Autodesk Inventor part; units mm, degrees
ref_plane "Arbeitsebene1" through (0, 4, 0) normal (0, 1, 0) x (-1, 0, 0)
ref_plane "YZ Plane" through (0, 0, 0) normal (1, 0, 0) x (0, 1, 0)
ref_plane "XZ Plane" through (0, 0, 0) normal (0, 1, 0) x (-1, 0, 0)
sketch "Skizze1" plane through (0, 0, 0) normal (0, 0, 1) x (1, 0, 0)
  circle A0 centre (0, 0) radius 4
  point P0 (0, 4)
  dimension "d0" = 8
extrude "Extrusion1" add sketch "Skizze1" along normal blind 15
ref_plane "Arbeitsebene1" through (0, 4, 0) normal (0, 1, 0) x (-1, 0, 0)
sketch "Skizze2" plane through (0, 4, 0) normal (0, 1, 0) x (-1, 0, 0)
  point P0 (0, 0)
  point P1 (0, 7.5)
  dimension "d3" = 7.5
hole "Bohrung1" at (0, 4, 7.5) direction (0, -1, 0) diameter 3.242 end through all
chamfer "Fase1" distance 1 angle 45 2 edges at (-4, 0, 0) (-4, 0, 15)
properties part number "LANGMUTTER"
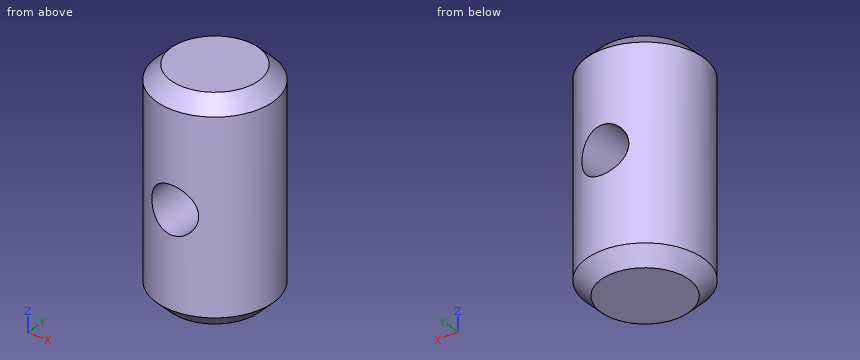
For this review, take the finished solid that the model builds, in its own axes (mm). Give positions to 0.01 mm unless a question says otherwise; leave off trailing zeros. Write each loop counter-clockwise with the first axis right and the second up, starting at its lowest first coordinate (ties: lowest second). Pieces come first, ordered by that corner, then holes. Notation, with made-up numbers: (-20, 66.5) -> (37, 66.5) arc R31 cw to (37, 91.5) -> close; hole circle Ø11 at (-13.75, 87.25). An arc over 180 degrees is marked (long way). Use CSV: the item, a comma, the result in double quotes.
Q1. To check wall thickness, follow probe 1 along Z at (x, y) = (0, -1.25); probe 2 along X at (y, z) = (-0.5, 7.5); probe 3 along Z at (x, y) = (1.25, 2). State the ranges of each line that lie inside material, in increasing order. Write a range as [from, to].
Conclusion:
probe 1,"[0, 5.88], [9.12, 15]"
probe 2,"[-3.97, -1.62], [1.62, 3.97]"
probe 3,"[0, 6.47], [8.53, 15]"
Q2. Take a section at C-C, the plane z = 6.5. Write out the cut boundary in (x, y).
Conclusion:
outline,"(-1.28, -3.79) -> (-1.28, 3.79) arc R4 ccw to start; (1.28, -3.79) arc R4 ccw to (1.28, 3.79) -> close"
Q3. Take a section at D-D, the plane z = 13.5. Write out the cut boundary in (x, y).
Conclusion:
outline,"circle Ø8 at (0, 0)"
Q4. For P1, Ø3, axis at y = -2, z = 13, coming from the +X side; P2, Ø2, axis at x = 2, z = 5, coming from the -Y side; P3, Ø1.5, axis at x = -3, z = 12.5, coming from the -Y side, all flat-tipped, find the tip position at first contact; note any pin that passes through.
Conclusion:
P1,"x = 3.97"
P2,"y = -3.87"
P3,"y = -3.31"
Q5. Take a section at B-B, the plane y = 0. Write out the cut boundary in (x, z), then the cut area to 3 significant figures.
Conclusion:
outline,"(-4, 1) -> (-3, 0) -> (3, 0) -> (4, 1) -> (4, 14) -> (3, 15) -> (-3, 15) -> (-4, 14) -> close; hole circle Ø3.24 at (0, 7.5)"
area,"110 mm2"
Q6. Take a section at A-A, the plane x = 0. Write out the cut boundary in (y, z), then the cut area to 3 significant figures.
Conclusion:
outline,"(-4, 1) -> (-3, 0) -> (3, 0) -> (4, 1) -> (4, 5.88) -> (-4, 5.88) -> close; (-4, 9.12) -> (4, 9.12) -> (4, 14) -> (3, 15) -> (-3, 15) -> (-4, 14) -> close"
area,"92.1 mm2"
